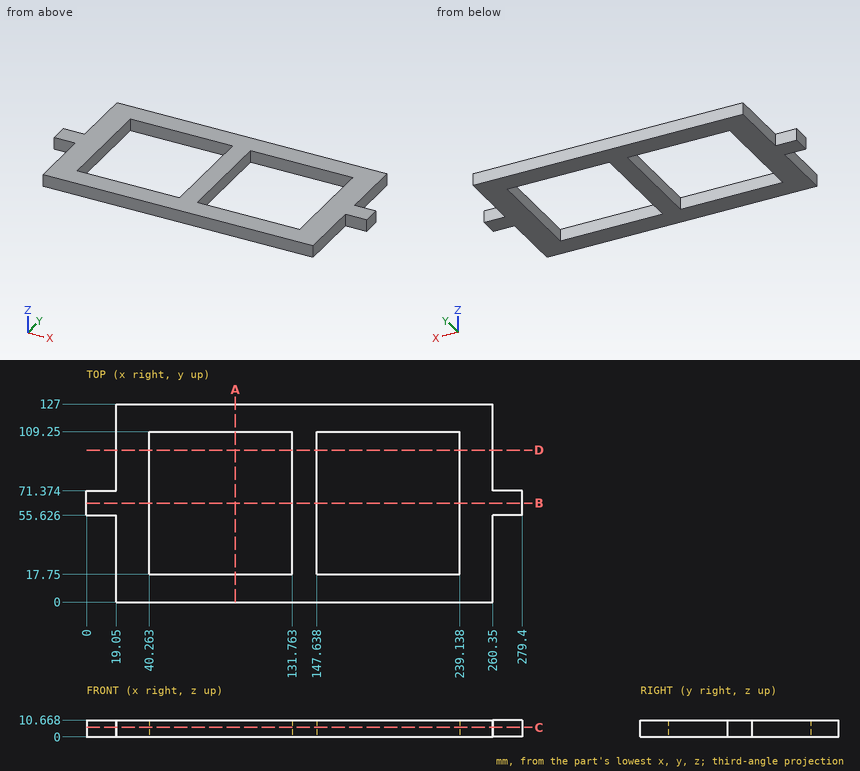
Study the drawing (mm; zero at the part's minimum x, y, z) and answer. Give positions to 0.01 mm unless a question says otherwise; leave off trailing zeros. Loops run counter-clockwise (first coordinate to the right, second up) from the corner with the lowest first, then second, coordinate; pieces in that order, holes last. Notation, with made-up numbers: M 20.25,23.25 L 58.25,23.25 A8 ccw 58.25,34.25 Z; hole C -32.75,3 d9. An arc over 180 degrees is marked long. One line per item, written item: value.
1. Section D-D on y = 97.5 is taken. Determine the outline of the cut face in (x, z).
Found:
outline: M 19.05,0 L 40.26,0 L 40.26,10.67 L 19.05,10.67 Z; M 131.76,0 L 147.64,0 L 147.64,10.67 L 131.76,10.67 Z; M 239.14,0 L 260.35,0 L 260.35,10.67 L 239.14,10.67 Z
2. Find the intervals of material crossed by probe 1 along X at (y, z) = (98.5, 2.75); probe 2 along X at (y, z) = (70, 4); probe 3 along Y at (x, z) = (207.5, 9), in increasing order.
Found:
probe 1: 19.05 to 40.26, 131.76 to 147.64, 239.14 to 260.35
probe 2: 0 to 40.26, 131.76 to 147.64, 239.14 to 279.4
probe 3: 0 to 17.75, 109.25 to 127
3. Section A-A on x = 95.5 is taken. Determine the outline of the cut face in (y, z), plus the area to 3 significant figures.
Found:
outline: M 0,0 L 17.75,0 L 17.75,10.67 L 0,10.67 Z; M 109.25,0 L 127,0 L 127,10.67 L 109.25,10.67 Z
area: 379 mm^2
4. Section B-B on y = 63.5 is taken. Determine the outline of the cut face in (x, z).
Found:
outline: M 0,0 L 40.26,0 L 40.26,10.67 L 0,10.67 Z; M 131.76,0 L 147.64,0 L 147.64,10.67 L 131.76,10.67 Z; M 239.14,0 L 279.4,0 L 279.4,10.67 L 239.14,10.67 Z
5. Each of these flat-tipped pins is pushed along its axis until it touches: P1, Ø5.5, axis at y = 84.5, z = 3, coming from the -X side; P2, Ø2, axis at y = 113, z = 4.5, coming from the +X side; P3, Ø5.5, axis at x = 271, z = 5.5, coming from the +Y side. Where does it stop, or does it pass through?
Found:
P1: x = 19.05
P2: x = 260.35
P3: y = 71.37
6. Section C-C on z = 6 is taken. State how many separate pieces and enclosed holes the cut face has, plus the area to 3 significant figures.
Found:
separate pieces: 1
enclosed holes: 2
area: 14,500 mm^2
